Design review of the part built by this model. Coordinates are the model's own, in mm. A direction names the side the tool comes from. Round coordinates to 2 decimals unless told otherwise and drop trailing zeros. Loops run counter-clockwise (first coordinate to the right, second up) from the corner with the lowest first, then second, coordinate; pieces in that order, holes last. Notation, with made-up numbers: (56.25, 68.25) - (107.25, 68.25) arc R30 cw to (107.25, 99.25) - close; hole circle Ø11 at (-37.75, 49). An arc over 180 degrees is marked (long way). Use one line per item in the form item = value. Start each with the question number.
(1) The part is to be moulded in two halves that separate along X. For faces 4 (the cylindrical face through (-14.274, -0.628, -0.056)), 5 (the cylindrical face through (-1.72, -7.75, 3.98)), 6 (the flat face through (6, -6, -4.762)), say which applies: released by +X, released by -X, zero draft, split by the parting line, or undercut.
(2) For pin 1 (3 mm diameter, centred on y = -6, z = -1, fed in from +X); pin 2 (1 mm diameter, centred on y = 3, z = -0.5, fed in from +X); pin 3 (1.5 mm diameter, centred on x = 10, z = 0, fed in from -Y), all flat-tipped, find the tip position at first contact; note any pin that passes through.
(3) We need section B-B, the plane z = 0. Write out the cut boundary in (x, y) (1 decimal).
(4) We need section A-A, the plane y = 0. Write out the cut boundary in (x, z) (1 decimal).
(5) Machinability: for faces 1 (the cylindrical face through (-1.72, -7.75, -3.96)), 2 (the flat face through (-8, 2, -3.175)), 3 (the cylindrical face through (13.358, -0.748, -2.374)), which of the approach directions +Z, -Z, +X, -X, +Y, -Y give a long, thin tool a straight path to every point of the face, cutting with its end or side? Answer none if there is none.
(6) Wall thickness on probe 1 along X at (y, z) = (-0.25, 3.5); probe 2 along Z at (x, y) = (-7.75, 7.5) (1 decimal); probe 3 along Y at (x, z) = (0, -1): over which ranges is each line inside the solid? List them lowest first. Write a range as [from, to].
(7) We need section C-C, the plane z = -1.5. Write out the cut boundary in (x, y) (1 decimal).
Autodesk Inventor part; units mm, degrees
ref_plane "Work Plane1" through (14.2875, 0, 0) normal (1, 0, 0) x (0, 1, 0)
ref_plane "XZ Plane" through (0, 0, 0) normal (0, 1, 0) x (-1, 0, 0)
ref_plane "XY Plane" through (0, 0, 0) normal (0, 0, 1) x (1, 0, 0)
sketch "Sketch1" plane through (0, 0, 0) normal (0, 0, 1) x (1, 0, 0)
  circle A0 centre (0, 0) radius 14.2875
  dimension "d0" = 28.575
extrude "Extrusion1" add sketch "Sketch1" along normal mid plane 9.525
fillet "Fillet1" radius 0.7937 2 edges at (-14.2875, 0, 4.7625) (-14.2875, 0, -4.7625)
sketch "Sketch2" plane through (0, 0, 4.7625) normal (0, 0, 1) x (1, 0, 0)
  circle A0 centre (0, 0) radius 13.4938
  circle A1 centre (0, 0) radius 7.9375
  dimension "d4" = 15.875
extrude "Extrusion2" cut sketch "Sketch2" against normal up to next contours A1
sketch "Sketch3" plane through (0, 0, 0) normal (1, 0, 0) x (0, 1, 0)
  line L0 (7.9375, 3.175) -> (11.9062, 3.175)
  line L1 (12.7, 2.3813) -> (12.7, -2.3813)
  line L2 (11.9062, -3.175) -> (7.9375, -3.175)
  line L3 (7.9375, -3.175) -> (7.9375, 3.175)
  line L4 (-13.4938, 4.7625) -> (13.4938, 4.7625)
  line L5 (13.4938, -4.7625) -> (-13.4938, -4.7625)
  line L6 (14.2875, -3.9688) -> (14.2875, 3.9688)
  line L7 (7.9375, 4.7625) -> (7.9375, -4.7625)
  arc A0 (12.7, 2.3813) -> (11.9062, 3.175) centre (11.9062, 2.3813) ccw
  arc A1 (11.9062, -3.175) -> (12.7, -2.3813) centre (11.9062, -2.3813) ccw
  line L8 (0, 4.7625) -> (0, -4.7625)
  point P0 (0, 0)
  dimension "d7" = 1.5875
  dimension "d8" = 1.5875
  dimension "d9" = 1.5875
  dimension "d10" = 0.7937
revolve "Revolution1" cut sketch "Sketch3" angle 360 about axis through (0, 0, 4.7625) along (0, 0, -1) contours L0 A0 L1 A1 L2 L3
ref_plane "Work Plane1" through (14.2875, 0, 0) normal (1, 0, 0) x (0, 1, 0)
sketch "Sketch4" plane through (14.2875, 0, 0) normal (1, 0, 0) x (0, 1, 0)
  line L0 (13.4938, -4.7625) -> (-13.4937, -4.7625)
  line L1 (14.2875, -3.9688) -> (14.2875, 3.9688)
  point P0 (0, 0)
  point P1 (0, 0)
hole "Hole1" at (14.2875, 0, 0) direction (-1, 0, 0) diameter 4.9784 depth 25.4 tip angle 118
equation "\"d8\" = d7"
equation "\"d9\" = d7"
properties part number "Misc_ShaftCollar_Triangle_SC10"
Data:
q1.face_4 = split by the parting line
q1.face_5 = undercut
q1.face_6 = zero draft
q2.pin_1 = 13.56
q2.pin_2 = 14.07
q2.pin_3 = -10.89
q3.outline = (12.5, -2.5) arc R12.7 cw (long way) to (12.5, 2.5) - (14.1, 2.5) arc R14.3 ccw (long way) to (14.1, -2.5) - close
q4.outline = (-14.3, -4) arc R0.8 ccw to (-13.5, -4.8) - (-7.9, -4.8) - (-7.9, -3.2) - (-11.9, -3.2) arc R0.8 cw to (-12.7, -2.4) - (-12.7, 2.4) arc R0.8 cw to (-11.9, 3.2) - (-7.9, 3.2) - (-7.9, 4.8) - (-13.5, 4.8) arc R0.8 ccw to (-14.3, 4) - close; (7.9, -4.8) - (13.5, -4.8) arc R0.8 ccw to (14.3, -4) - (14.3, -2.5) - (12.7, -2.5) arc R0.8 cw to (11.9, -3.2) - (7.9, -3.2) - close; (7.9, 3.2) - (11.9, 3.2) arc R0.8 cw to (12.7, 2.5) - (14.3, 2.5) - (14.3, 4) arc R0.8 ccw to (13.5, 4.8) - (7.9, 4.8) - close
q5.face_1 = +Z, -Z
q5.face_2 = none
q5.face_3 = +X
q6.probe_1 = [-14.29, -7.93], [7.93, 14.29]
q6.probe_2 = [-4.8, -3.2], [3.2, 4.8]
q6.probe_3 = [-14.29, -12.7], [12.7, 14.29]
q7.outline = (12.5, -2) arc R12.7 cw (long way) to (12.5, 2) - (14.1, 2) arc R14.3 ccw (long way) to (14.1, -2) - close
